```python
from build123d import *

# Parameters (mm, degrees)
SKETCH2_R      = 0.5
F_0TO0_5_DEPTH = 6.349
SKETCH3_R      = 1
SKETCH3_R_2    = 0.5
F_0_5TO1_DEPTH = 6.351
SKETCH4_R      = 1.5
SKETCH4_R_2    = 1
F_1TO1_5_DEPTH = 6.349
SKETCH5_R      = 2
SKETCH5_R_2    = 1.5
F_1_5TO2_DEPTH = 6.351
SKETCH6_R      = 2.5
SKETCH6_R_2    = 2
F_2TO2_5_DEPTH = 6.349
SKETCH7_R      = 3
SKETCH7_R_2    = 2.5
F_2_5TO3_DEPTH = 6.351
SKETCH8_R      = 6.5
MIRROR_2_DEPTH = 6.35


with BuildPart() as part:
    # Sketch2 → 0to0.5 (new body)
    with BuildSketch(Plane.XY):
        Circle(SKETCH2_R)
    extrude(amount=F_0TO0_5_DEPTH)

    # Sketch3 → 0.5to1 (add)
    with BuildSketch(Plane.XY):
        Circle(SKETCH3_R)
        Circle(SKETCH3_R_2, mode=Mode.SUBTRACT)
    extrude(amount=F_0_5TO1_DEPTH)

    # Sketch4 → 1to1.5 (add)
    with BuildSketch(Plane.XY):
        Circle(SKETCH4_R)
        Circle(SKETCH4_R_2, mode=Mode.SUBTRACT)
    extrude(amount=F_1TO1_5_DEPTH)

    # Sketch5 → 1.5to2 (add)
    with BuildSketch(Plane.XY):
        Circle(SKETCH5_R)
        Circle(SKETCH5_R_2, mode=Mode.SUBTRACT)
    extrude(amount=F_1_5TO2_DEPTH)

    # Sketch6 → 2to2.5 (add)
    with BuildSketch(Plane.XY):
        Circle(SKETCH6_R)
        Circle(SKETCH6_R_2, mode=Mode.SUBTRACT)
    extrude(amount=F_2TO2_5_DEPTH)

    # Sketch7 → 2.5to3 (add)
    with BuildSketch(Plane.XY):
        Circle(SKETCH7_R)
        Circle(SKETCH7_R_2, mode=Mode.SUBTRACT)
    extrude(amount=F_2_5TO3_DEPTH)

    # Sketch8 → Mirror 2 (add)
    with BuildSketch(Plane.XY):
        Circle(SKETCH8_R)
    extrude(amount=MIRROR_2_DEPTH)


solid = part.part
```
Input: part model. Units: mm. Frame: model coordinates. Give positions to 0.01 mm unless a question says otherwise; leave off trailing zeros. Loops run counter-clockwise (first coordinate to the right, second up) from the corner with the lowest first, then second, coordinate; pieces in that order, holes last. Notation, with made-up numbers: (74, -3.75) -> (121, -3.75) arc R13 cw to (121, 13.25) -> close; hole circle Ø5 at (-4.75, -30). An arc over 180 degrees is marked (long way). Use a Markdown table: item, result.
Q1. Section query B-B, the plane z = 1.5. Return the cut outline in (x, y), plus the area to 3 significant figures.
Entries:
| item | result |
|---|---|
| outline | circle Ø13 at (0, 0) |
| area | 133 mm² |
Q2. First-contact query: P1, Ø3, axis at y = 5, z = 4.5, coming from the +X side; P2, Ø1, axis at y = 5, z = 2.5, coming from the +X side; P3, Ø1.5, axis at y = -5, z = 4.5, coming from the -X side. Flat tips, straight axial feed; report the tip coordinate or a pass-through.
Entries:
| item | result |
|---|---|
| P1 | stops at x = 5.48 |
| P2 | stops at x = 4.69 |
| P3 | stops at x = -4.92 |
Q3. Section query D-D, the plane y = -5.5. Return the cut outline in (x, z).
Entries:
| item | result |
|---|---|
| outline | (-3.46, 0) -> (3.46, 0) -> (3.46, 6.35) -> (-3.46, 6.35) -> close |
Q4. Section query C-C, the plane y = 5.75. Return the cut outline in (x, z).
Entries:
| item | result |
|---|---|
| outline | (-3.03, 0) -> (3.03, 0) -> (3.03, 6.35) -> (-3.03, 6.35) -> close |
Q5. Ray query, probe 1 along Z at (x, y) = (6.25, 1.5); probe 2 along Y at (x, z) = (6, 2); probe 3 along Y at (x, z) = (1.25, 6). Return the intervals inside material, ascending. Write a range as from..to.
Entries:
| item | result |
|---|---|
| probe 1 | z = 0..6.35 |
| probe 2 | y = -2.5..2.5 |
| probe 3 | y = -6.38..6.38 |
